For this review, take the finished solid that the model builds, in its own axes (mm). A direction names the side the tool comes from. Coordinates: 2 decimals unless noted, no trailing zeros. Order: outer loops, then holes, each group sorted by start corner. A loop starts at its lowest first (then second) coordinate and runs counter-clockwise, first axis right, second up. Notation, with made-up numbers: (75.25, 77) -> (121.25, 77) arc R31 ccw to (121.25, 108) -> close; hole circle Ø1 at (-37, 41). An arc over 180 degrees is marked (long way). Answer as a JSON object with one key per item and string values. Group by question number.
1) Wall thickness on L1, parallel to Y at x = 5, z = -2; L2, parallel to X at y = 42.5, z = -11; L3, parallel to Z at x = 37, y = 6: over which ranges is each line inside the solid? List them lowest first.
2) Add section A-A, the plane y = 52. Write out the cut boundary in (x, z).
3) Machinability: for faces 5 (the cylindrical face through (46.23, 46.16, -60.25)), 6 (the cylindrical face through (44.6, 1.9, -60.2)), 7 (the cylindrical face through (41.4, 84.1, -60.2)), 8 (the cylindrical face through (84.22, 41.574, -60.249)), 9 (the cylindrical face through (1.78, 44.426, -60.249)), which of the approach directions +Z, -Z, +X, -X, +Y, -Y give a long, thin tool a straight path to every point of the face, cutting with its end or side? Answer none if there is none.
4) Add section C-C, the plane z = -91. Write out the cut boundary in (x, y), then the cut area to 3 significant figures.
5) For pin 1 (5 mm diameter, centred on x = 18.5, y = 20.5, fed in from -Z); pin 2 (6 mm diameter, centred on y = 50.5, z = -42, fed in from -X); pin 3 (3 mm diameter, centred on x = 48, z = -72.5, fed in from +Y), all flat-tipped, find the tip position at first contact; note any pin that passes through.
6) Add section D-D, the plane x = 21.5. Write out the cut boundary in (y, z), then the cut area to 3 significant figures.
7) Draft analysis for pull direction X (two halves, no side actions). For faces 1 (the cylindrical face through (54.31, 51.04, -2.96)), 2 (the cylindrical face through (7.385, 5.751, -2.958)), 3 (the flat face through (0, 43, -39)), 4 (the flat face through (43, 43, -113)), state which applies: +X half, -X half, draft (parallel to the pull), parting line (faces both ways), or undercut.
Autodesk Inventor part; units mm, degrees
ref_plane "YZ Plane" through (0, 0, 0) normal (1, 0, 0) x (0, 1, 0)
ref_plane "XZ Plane" through (0, 0, 0) normal (0, 1, 0) x (-1, 0, 0)
sketch "Sketch1" plane through (0, 0, 0) normal (0, 0, 1) x (1, 0, 0)
  line L0 (0, 0) -> (86, 0)
  line L1 (86, 0) -> (86, 86)
  line L2 (86, 86) -> (0, 86)
  line L3 (0, 86) -> (0, 0)
  circle A0 centre (5, 5) radius 2.5
  circle A1 centre (52, 5) radius 2.5
  circle A2 centre (5, 52) radius 2.5
  circle A3 centre (52, 52) radius 2.5
  dimension "d0" = 86
  dimension "d1" = 86
  dimension "d2" = 5
  dimension "d3" = 5
  dimension "d4" = 5
extrude "Extrusion1" add sketch "Sketch1" against normal blind 113
sketch "Sketch2" plane through (0, 0, -113) normal (0, 0, -1) x (-1, 0, 0)
  line L0 (0, 86) -> (-86, 86)
  line L1 (-43, 86) -> (-43, 0)
  line L2 (-86, 0) -> (0, 0)
  line L3 (-86, 86) -> (-86, 0)
  line L4 (-86, 43) -> (0, 43)
  line L5 (0, 0) -> (0, 86)
  arc A0 (-46.3441, 0) -> (-86, 39.9524) centre (-66.1721, 19.9762) ccw
  line L6 (-86, 39.9524) -> (-86, 0)
  line L7 (0, 0) -> (-86, 0)
  line L8 (0, 86) -> (0, 0)
  arc A1 (0, 39.9524) -> (-39.6559, 0) centre (-19.8279, 19.9762) ccw
  line L9 (-86, 86) -> (0, 86)
  arc A2 (-86, 46.0476) -> (-46.3441, 86) centre (-66.1721, 66.0238) ccw
  line L10 (-86, 46.0476) -> (-86, 86)
  arc A3 (-39.6559, 86) -> (0, 46.0476) centre (-19.8279, 66.0238) ccw
  line L11 (0, 86) -> (-86, 86)
  point P0 (0, 39.9524)
  point P1 (-39.6559, 0)
  point P2 (-39.6559, 86)
  point P3 (0, 46.0476)
  point P4 (-86, 46.0476)
  point P5 (-46.3441, 86)
extrude "Extrusion2" cut sketch "Sketch2" against normal blind 107 contours L5 A3 A1 A2 L0 | A2 L1 | A3 A2 A0 L3 L0 | L1 A3 | A3 L4 | L4 A1 | A1 L5 L2 A0 A3 | A2 L4 | L4 A0 | A0 A1 L2 L3 A2 | A0 L1 | L1 A1
properties part number "nema34"
Output values:
{
 "1": {"L1": "y = 0 to 2.5, 7.5 to 49.5, 54.5 to 86", "L2": "x = 0 to 2.95, 36.71 to 49.29, 83.05 to 86", "L3": "z = -6 to 0"},
 "2": {"outline": "(0, -6) -> (2.5, -6) -> (2.5, 0) -> (0, 0) -> close; (7.5, -6) -> (49.5, -6) -> (49.5, 0) -> (7.5, 0) -> close; (54.5, -6) -> (86, -6) -> (86, 0) -> (54.5, 0) -> close"},
 "3": {"face 5": "-Z", "face 6": "-Z, +X", "face 7": "-Z, -X", "face 8": "-Z, -Y", "face 9": "-Z, +Y"},
 "4": {"outline": "(0, 39.95) arc R28.15 cw to (3.64, 43) arc R28.15 cw to (0, 46.05) -> close; (36.02, 43) arc R28.15 cw to (43, 35.95) arc R28.15 cw to (49.98, 43) arc R28.15 cw to (43, 50.05) arc R28.15 cw to start; (39.66, 0) -> (46.34, 0) arc R28.15 cw to (43, 4) arc R28.15 cw to start; (39.66, 86) arc R28.15 cw to (43, 82) arc R28.15 cw to (46.34, 86) -> close; (82.36, 43) arc R28.15 cw to (86, 39.95) -> (86, 46.05) arc R28.15 cw to start", "area": "133 mm²"},
 "5": {"pin 1": "stops at z = -6", "pin 2": "stops at x = 41.02", "pin 3": "stops at y = 45.89"},
 "6": {"outline": "(0, -6) -> (86, -6) -> (86, 0) -> (0, 0) -> close", "area": "516 mm²"},
 "7": {"face 1": "undercut", "face 2": "undercut", "face 3": "-X half", "face 4": "draft"}
}
